The model under review builds one solid part; all positions refer to its coordinate system, in mm. A direction names the side the tool comes from. Coordinates: 2 decimals unless noted, no trailing zeros. Loops run counter-clockwise (first coordinate to the right, second up) from the corner with the lowest first, then second, coordinate; pieces in that order, holes last. Notation, with made-up numbers: (-2.75, 71) -> (21.25, 71) arc R22 cw to (21.25, 90) -> close; hole circle Ø5 at (40, 15). An arc over 180 degrees is marked (long way). One line per question, with ' | ' between items. Start each with the question number.
from build123d import *

# Parameters (mm, degrees)
SKETCH_1_W          = 40
SKETCH_1_H          = 39
EXTRUDE_2_DEPTH     = 20
FILLET_2_R          = 0.5
FILLET_3_R          = 0.5
FILLET_4_R          = 0.5
FILLET_5_R          = 0.5
SKETCH_6_W          = 19
SKETCH_6_H          = 2
EXTRUDE_3_DEPTH     = 8
SKETCH_7_W          = 19
SKETCH_7_H          = 2
EXTRUDE_5_DEPTH     = 8
SKETCH_8_R          = 2
CUT_EXTRUDE_1_DEPTH = 28
SKETCH_9_R          = 6
SKETCH_9_R_2        = 4.5
EXTRUDE_7_DEPTH     = 1
SKETCH_10_R         = 4.5
EXTRUDE_8_DEPTH     = 1.5
SKETCH_11_R         = 3
EXTRUDE_9_DEPTH     = 4.5
SKETCH_12_R         = 1.5
CUT_EXTRUDE_2_DEPTH = 6


with BuildPart() as part:
    # 草图1 → 凸台-拉伸2 (new body)
    with BuildSketch(Plane.XY):
        with Locations((20, 19.5)):
            Rectangle(SKETCH_1_W, SKETCH_1_H)
    extrude(amount=EXTRUDE_2_DEPTH)

    # 圆角2
    fillet_2_edges = [part.edges().sort_by_distance(p)[0] for p in [
        (40, 19.5, 20),
        (20, 39, 20),
    ]]
    fillet(fillet_2_edges, radius=FILLET_2_R)

    # 圆角3
    fillet_3_edges = [part.edges().sort_by_distance(p)[0] for p in [
        (40, 0, 9.75),
        (19.75, 0, 20),
        (39.853553391, 0, 19.853553391),
        (0, 39, 9.75),
        (0, 38.853553391, 19.853553391),
        (0, 19.25, 20),
    ]]
    fillet(fillet_3_edges, radius=FILLET_3_R)

    # 圆角4
    # the kernel refuses this fillet: 0.5 mm, written as the material it takes off along each edge
    with BuildSketch(Plane(origin=(39.5, 38.5, 19.5), x_dir=(0, 1, 0), z_dir=(1, 0, 0))) as fillet_4_piece_1_section:
        Polygon((0, 0), (FILLET_4_R, 0), (FILLET_4_R, FILLET_4_R), (0, FILLET_4_R), align=None)
    fillet_4_piece_1 = extrude(amount=FILLET_4_R, mode=Mode.PRIVATE)
    fillet_4_piece_1 = fillet_4_piece_1 - Plane(origin=(39.5, 38.5, 19.5), x_dir=(0, -0.7071067811865475, -0.7071067811865475), z_dir=(1, 0, 0)) * Sphere(FILLET_4_R, mode=Mode.PRIVATE)
    add(fillet_4_piece_1, mode=Mode.SUBTRACT)
    with BuildSketch(Plane(origin=(40, 39, -1.25), x_dir=(0, -1, 0), z_dir=(0, 0, 1))) as fillet_4_piece_2:
        with BuildLine():
            CenterArc((FILLET_4_R, -FILLET_4_R), FILLET_4_R, 90, 90)
            Line((0, -FILLET_4_R), (0, 0))
            Line((0, 0), (FILLET_4_R, 0))
        make_face()
    extrude(amount=20.75, mode=Mode.SUBTRACT)
    with BuildSketch(Plane(origin=(40, 0.5, 0), x_dir=(-1, 0, 0), z_dir=(0, 1, 0))) as fillet_4_piece_3:
        with BuildLine():
            CenterArc((FILLET_4_R, FILLET_4_R), FILLET_4_R, 180, 90)
            Line((0, FILLET_4_R), (0, 0))
            Line((0, 0), (FILLET_4_R, 0))
        make_face()
    extrude(amount=39.75, mode=Mode.SUBTRACT)
    with BuildSketch(Plane(origin=(39.5, 0.5, 0), x_dir=(0, -1, 0), z_dir=(-1, 0, 0))) as fillet_4_piece_4:
        with BuildLine():
            CenterArc((0.5 - FILLET_4_R, FILLET_4_R), FILLET_4_R, 270, 90)
            Line((0.5, FILLET_4_R), (0.5, 0))
            Line((0.5, 0), (0.5 - FILLET_4_R, 0))
        make_face()
    revolve(axis=Axis((39.5, 0.5, 0), (0, 0, 1)), revolution_arc=90, mode=Mode.SUBTRACT)
    with BuildSketch(Plane(origin=(-1.25, 0, 0), x_dir=(0, 0, 1), z_dir=(1, 0, 0))) as fillet_4_piece_5:
        with BuildLine():
            CenterArc((FILLET_4_R, -FILLET_4_R), FILLET_4_R, 90, 90)
            Line((0, -FILLET_4_R), (0, 0))
            Line((0, 0), (FILLET_4_R, 0))
        make_face()
    extrude(amount=40.75, mode=Mode.SUBTRACT)

    # 圆角5
    # the kernel refuses this fillet: 0.5 mm, written as the material it takes off along each edge
    with BuildSketch(Plane(origin=(0.5, 0.5, 19.5), x_dir=(-1, 0, 0), z_dir=(0, -1, 0))) as fillet_5_piece_1_section:
        Polygon((0, 0), (FILLET_5_R, 0), (FILLET_5_R, -FILLET_5_R), (0, -FILLET_5_R), align=None)
    fillet_5_piece_1 = extrude(amount=FILLET_5_R, mode=Mode.PRIVATE)
    fillet_5_piece_1 = fillet_5_piece_1 - Plane(origin=(0.5, 0.5, 19.5), x_dir=(0.7071067811865475, 0, -0.7071067811865475), z_dir=(0, -1, 0)) * Sphere(FILLET_5_R, mode=Mode.PRIVATE)
    add(fillet_5_piece_1, mode=Mode.SUBTRACT)
    with BuildSketch(Plane(origin=(39.5, 38.5, 0.5), x_dir=(0, 1, 0), z_dir=(0, 0, -1))) as fillet_5_piece_2_section:
        Polygon((0, 0), (FILLET_5_R, 0), (FILLET_5_R, FILLET_5_R), (0, FILLET_5_R), align=None)
    fillet_5_piece_2 = extrude(amount=FILLET_5_R, mode=Mode.PRIVATE)
    fillet_5_piece_2 = fillet_5_piece_2 - Plane(origin=(39.5, 38.5, 0.5), x_dir=(-0.7071067811865475, -0.7071067811865477, 0), z_dir=(0, 0, -1)) * Sphere(FILLET_5_R, mode=Mode.PRIVATE)
    add(fillet_5_piece_2, mode=Mode.SUBTRACT)
    with BuildSketch(Plane(origin=(39.5, 39, 0), x_dir=(0, -1, 0), z_dir=(-1, 0, 0))) as fillet_5_piece_3:
        with BuildLine():
            CenterArc((FILLET_5_R, FILLET_5_R), FILLET_5_R, 180, 90)
            Line((0, FILLET_5_R), (0, 0))
            Line((0, 0), (FILLET_5_R, 0))
        make_face()
    extrude(amount=39, mode=Mode.SUBTRACT)
    with BuildSketch(Plane(origin=(0.5, 38.5, 0), x_dir=(-1, 0, 0), z_dir=(0, -1, 0))) as fillet_5_piece_4:
        with BuildLine():
            CenterArc((0.5 - FILLET_5_R, -FILLET_5_R), FILLET_5_R, 0, 90)
            Line((0.5, -FILLET_5_R), (0.5, 0))
            Line((0.5, 0), (0.5 - FILLET_5_R, 0))
        make_face()
    revolve(axis=Axis((0.5, 38.5, 0), (0, 0, -1)), revolution_arc=90, mode=Mode.SUBTRACT)
    with BuildSketch(Plane(origin=(0, 0, 0.5), x_dir=(1, 0, 0), z_dir=(0, 0, 1))) as fillet_5_piece_5:
        with BuildLine():
            CenterArc((FILLET_5_R, FILLET_5_R), FILLET_5_R, 180, 90)
            Line((0, FILLET_5_R), (0, 0))
            Line((0, 0), (FILLET_5_R, 0))
        make_face()
    extrude(amount=19, mode=Mode.SUBTRACT)
    with BuildSketch(Plane(origin=(0, 38.5, 0), x_dir=(0, 0, 1), z_dir=(0, -1, 0))) as fillet_5_piece_6:
        with BuildLine():
            CenterArc((FILLET_5_R, -FILLET_5_R), FILLET_5_R, 90, 90)
            Line((0, -FILLET_5_R), (0, 0))
            Line((0, 0), (FILLET_5_R, 0))
        make_face()
    extrude(amount=38, mode=Mode.SUBTRACT)
    with BuildSketch(Plane(origin=(0, 0.5, 0.5), x_dir=(0, 0, -1), z_dir=(0, 1, 0))) as fillet_5_piece_7:
        with BuildLine():
            CenterArc((0.5 - FILLET_5_R, -FILLET_5_R), FILLET_5_R, 0, 90)
            Line((0.5 - FILLET_5_R, 0), (0.5, 0))
            Line((0.5, 0), (0.5, -FILLET_5_R))
        make_face()
    revolve(axis=Axis((0, 0.5, 0.5), (-1, 0, 0)), revolution_arc=90, mode=Mode.SUBTRACT)

    # 草图6 → 凸台-拉伸3 (add)
    with BuildSketch(Plane.ZY):
        with Locations((10, 30)):
            Rectangle(SKETCH_6_W, SKETCH_6_H)
    extrude(amount=EXTRUDE_3_DEPTH)

    # 草图7 → 凸台-拉伸5 (add)
    with BuildSketch(Plane(origin=(40, 0, 0), x_dir=(0, 0, -1), z_dir=(1, 0, 0))):
        with Locations((-10, 30)):
            Rectangle(SKETCH_7_W, SKETCH_7_H)
    extrude(amount=EXTRUDE_5_DEPTH)

    # 草图8 → 切除-拉伸1 (cut)
    with BuildSketch(Plane(origin=(0, 39, 0), x_dir=(1, 0, 0), z_dir=(0, 1, 0))):
        with Locations(Location((-3.928154272, -5, 0), (0, 0, 180))):
            Circle(SKETCH_8_R)
        with Locations(Location((-3.928154272, -15, 0), (0, 0, 180))):
            Circle(SKETCH_8_R)
        with Locations(Location((44.071845728, -5, 0), (0, 0, 180))):
            Circle(SKETCH_8_R)
        with Locations(Location((44.071845728, -15, 0), (0, 0, 180))):
            Circle(SKETCH_8_R)
    extrude(amount=-CUT_EXTRUDE_1_DEPTH, mode=Mode.SUBTRACT)

    # 草图9 → 凸台-拉伸7 (add)
    with BuildSketch(Plane(origin=(0, 39, 0), x_dir=(1, 0, 0), z_dir=(0, 1, 0))):
        with Locations(Location((10.071845728, -10.288024079, 0), (0, 0, 270))):
            Circle(SKETCH_9_R)
        with Locations(Location((10.071845728, -10.288024079, 0), (0, 0, 270))):
            Circle(SKETCH_9_R_2, mode=Mode.SUBTRACT)
    extrude(amount=EXTRUDE_7_DEPTH)

    # 草图10 → 凸台-拉伸8 (add)
    with BuildSketch(Plane(origin=(0, 39, 0), x_dir=(1, 0, 0), z_dir=(0, 1, 0))):
        with Locations(Location((10.071845728, -10.288024079, 0), (0, 0, 270))):
            Circle(SKETCH_10_R)
    extrude(amount=EXTRUDE_8_DEPTH)

    # 草图11 → 凸台-拉伸9 (add)
    with BuildSketch(Plane(origin=(0, 40.5, 0), x_dir=(1, 0, 0), z_dir=(0, 1, 0))):
        with Locations(Location((10.071845728, -10.288024079, 0), (0, 0, 270))):
            Circle(SKETCH_11_R)
    extrude(amount=EXTRUDE_9_DEPTH)

    # 草图12 → 切除-拉伸2 (cut)
    with BuildSketch(Plane(origin=(0, 45, 0), x_dir=(1, 0, 0), z_dir=(0, 1, 0))):
        with Locations(Location((10.071845728, -10.288024079, 0), (0, 0, 270))):
            Circle(SKETCH_12_R)
    extrude(amount=-CUT_EXTRUDE_2_DEPTH, mode=Mode.SUBTRACT)


solid = part.part
1) Machinability: for faces 5 (the face through (44, 30, 19.5)), 6 (the face through (44, 29, 10)), 7 (the face through (14.13, 39.49, 5.87)), 8 (the face through (40, 35, 10)), 9 (the face through (0, 15, 10)), which of the approach directions +Z, -Z, +X, -X, +Y, -Y give a long, thin tool a straight path to every point of the face, cutting with its end or side? Answer none if there is none.
2) Insertion check: pin 1 Ø6 at (x, z) = (4, 5) entering from +Y; pin 2 Ø2 at (y, z) = (34, 6.5) entering from -X; pin 3 Ø1 at (x, y) = (-2, 30) entering from +Z; pin 4 Ø3 at (x, y) = (35.5, 15.5) entering from -Z. Each pin has a flat end and moves straight along its axis. Give the tip position at first contact, or say it passes through.
3) Consider section B-B, the plane x = 35.5. Write out the cut boundary in (y, z).
4) Wall thickness on L1, parallel to X at y = 21, z = 5.25; L2, parallel to Y at x = 4, z = 9.25; L3, parallel to Y at x = -1, z = 17.75: over which ranges is each line inside the solid? List them lowest first.
5) Consider section A-A, the plane z = 5. Write out the cut boundary in (x, y), plus the area to 3 significant figures.
6) Mouldability with a two-part tool opening along Z and no side actions: class faces 1 (the face through (-4, 30, 19.5)), 2 (the face through (9.497, 42.042, 11.674)), 3 (the face through (-4, 31, 10)), 4 (the face through (44, 30, 0.5)) as +Z half, -Z half, draft (parallel to the pull), parting line (faces both ways), or undercut.
7) Consider section C-C, the plane y = 25. Write out the cut boundary in (x, z).
Filled sheet:
1) face 5: +Z, +X, +Y, -Y | face 6: +Z, -Z, +X, -Y | face 7: +Y | face 8: +Z, -Z, +X, +Y | face 9: +Z, -Z, -X, -Y
2) pin 1: y = 40 | pin 2: x = 0 | pin 3: z = 19.5 | pin 4: z = 0
3) outline: (0, 0.5) arc R0.5 ccw to (0.5, 0) -> (38.5, 0) arc R0.5 ccw to (39, 0.5) -> (39, 19.5) arc R0.5 ccw to (38.5, 20) -> (0.5, 20) arc R0.5 ccw to (0, 19.5) -> close
4) L1: 0 to 40 | L2: 0 to 39 | L3: 29 to 31
5) outline: (-8, 29) -> (-5.93, 29) -> (-5.93, 31) -> (-8, 31) -> close; (-1.93, 29) -> (0, 29) -> (0, 0.5) arc R0.5 ccw to (0.5, 0) -> (39.5, 0) arc R0.5 ccw to (40, 0.5) -> (40, 29) -> (42.07, 29) -> (42.07, 31) -> (40, 31) -> (40, 38.5) arc R0.5 ccw to (39.5, 39) -> (12.91, 39) -> (12.91, 40) -> (7.24, 40) -> (7.24, 39) -> (0.5, 39) arc R0.5 ccw to (0, 38.5) -> (0, 31) -> (-1.93, 31) -> close; (46.07, 29) -> (48, 29) -> (48, 31) -> (46.07, 31) -> close | area: 1,580 mm^2
6) face 1: +Z half | face 2: undercut | face 3: draft | face 4: -Z half
7) outline: (0, 0.5) arc R0.5 ccw to (0.5, 0) -> (39.5, 0) arc R0.5 ccw to (40, 0.5) -> (40, 19.5) arc R0.5 ccw to (39.5, 20) -> (0.5, 20) arc R0.5 ccw to (0, 19.5) -> close
